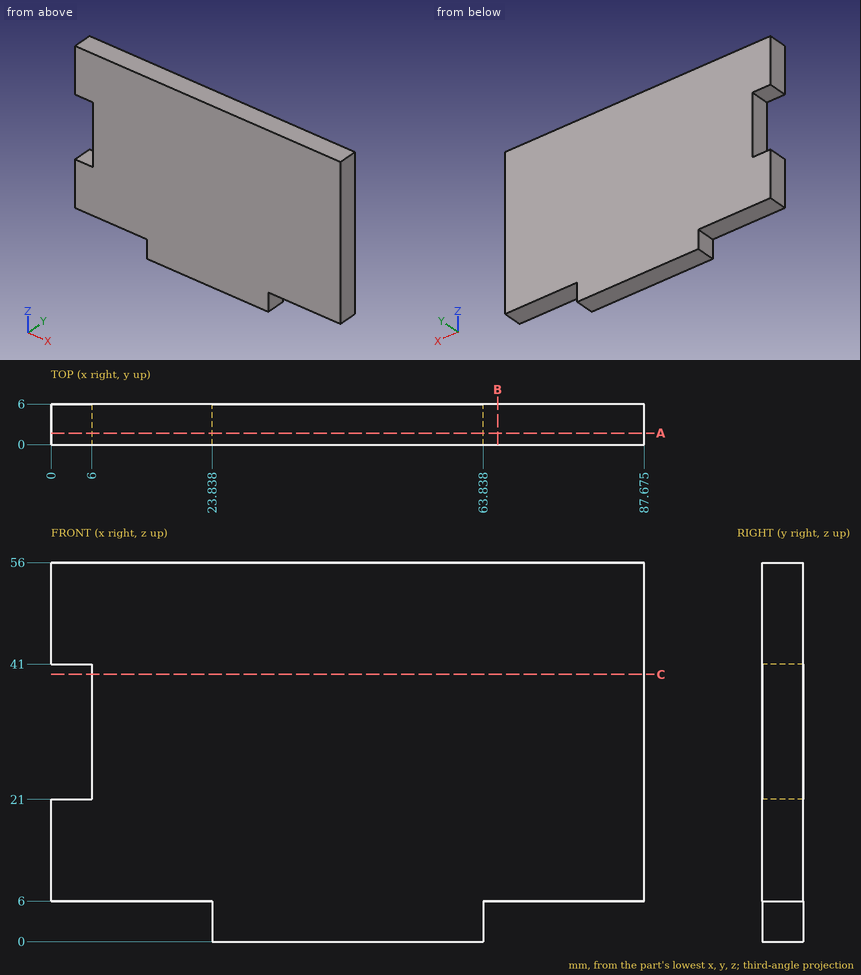
Geometry check sheet. Reference: drawing and pictorial views, mm from the part's lowest x, y, z. Coordinates: 2 decimals unless noted, no trailing zeros. Write each loop counter-clockwise with the first axis right and the second up, starting at its lowest first coordinate (ties: lowest second). Pieces come first, ordered by that corner, then holes. Notation, with made-up numbers: (75.5, 4.25) - (108.5, 4.25) arc R24 ccw to (108.5, 38.25) - close; hole circle Ø5 at (-15.5, 81.5). An arc over 180 degrees is marked (long way). Write item = value, one per line.
Q1. Cross-section at B-B (x = 66). Enter the section's corners in (y, z), plus the area to 3 significant figures.
Answer:
outline = (0, 6) - (6, 6) - (6, 56) - (0, 56) - close
area = 300 mm²
Q2. Material ranges on L1, parallel to Z at x = 78.5, y = 3.3; L2, parallel to X at y = 5.2, z = 28.5 (1 decimal); L3, parallel to X at y = 4.45, z = 5, recorded low to high. Write a range as from..to.
Answer:
L1 = 6..56
L2 = 6..87.7
L3 = 23.84..63.84
Q3. Cross-section at A-A (y = 1.7). Enter the section's corners in (x, z) (1 decimal).
Answer:
outline = (0, 6) - (23.8, 6) - (23.8, 0) - (63.8, 0) - (63.8, 6) - (87.7, 6) - (87.7, 56) - (0, 56) - (0, 41) - (6, 41) - (6, 21) - (0, 21) - close
Q4. Go/stop test with flat-tipped pins: pin 1 Ø3 at (x, y) = (53.5, 1) entering from -Z; pin 2 Ø3 at (x, y) = (80, 2) entering from -Z; pin 3 Ø3 at (y, z) = (2, 2) entering from +X; pin 4 Ø1.8 at (y, z) = (3, 3) entering from -X. Record where each tip stops, or that it passes through.
Answer:
pin_1 = 0
pin_2 = 6
pin_3 = 63.84
pin_4 = 23.84
Q5. Cross-section at C-C (z = 39.5). Enter the section's corners in (x, y) (1 decimal).
Answer:
outline = (6, 0) - (87.7, 0) - (87.7, 6) - (6, 6) - close
